Geometry check sheet. Reference: the model listing, model coordinates, mm. Face numbers are marked on the shaded views. A direction names the side the tool comes from. Give positions to 0.01 mm unless a question says otherwise; leave off trailing zeros. Loops run counter-clockwise (first coordinate to the right, second up) from the corner with the lowest first, then second, coordinate; pieces in that order, holes last. Notation, with made-up numbers: (-22, 44.5) -> (37, 44.5) arc R18 ccw to (37, 74.5) -> close; hole circle Ø1 at (54, 16). An arc over 180 degrees is marked (long way). Write item = value, one per line.
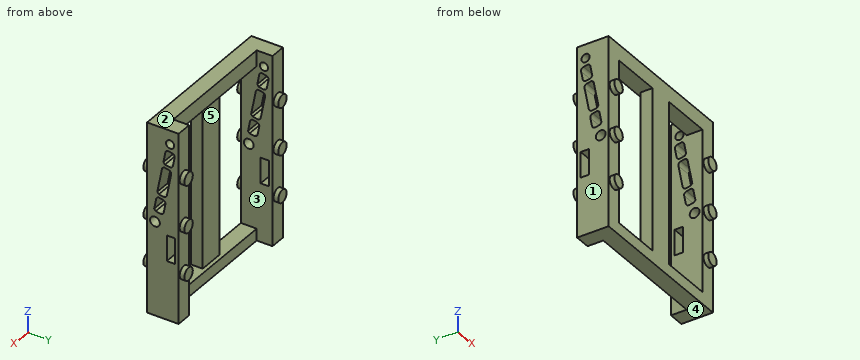
```python
from build123d import *

# Parameters (mm, degrees)
SKETCH1_W               = 100
SKETCH1_H               = 120
SKETCH1_W_2             = 80
SKETCH1_H_2             = 102.5
BOSS_EXTRUDE1_DEPTH     = 20
SKETCH2_R               = 4
BOSS_EXTRUDE2_DEPTH     = 3
MIRROR2_COPY_1_SKETCH_R = 4
MIRROR2_COPY_1_DEPTH    = 3
SKETCH8_W               = 80
SKETCH8_H               = 10
CUT_EXTRUDE5_DEPTH      = 133.018938035
SKETCH12_R              = 3.1
SKETCH12_R_2            = 2.6
CUT_EXTRUDE7_DEPTH      = 14
SKETCH15_W              = 16
SKETCH15_H              = 7.5
BOSS_EXTRUDE4_DEPTH     = 102.5
SKETCH18_W              = 16.2
SKETCH18_H              = 5.2
CUT_EXTRUDE10_DEPTH     = 119.865470175


with BuildPart() as part:
    # Sketch1 → Boss-Extrude1 (new body)
    with BuildSketch(Plane(origin=(0, 0, 0), x_dir=(1, 0, 0), z_dir=(0, 1, 0))):
        Rectangle(SKETCH1_W, SKETCH1_H)
        with Locations((0, 1.25)):
            Rectangle(SKETCH1_W_2, SKETCH1_H_2, mode=Mode.SUBTRACT)
    extrude(amount=BOSS_EXTRUDE1_DEPTH)

    # Sketch2 → Boss-Extrude2 (add)
    with BuildSketch(Plane(origin=(0, 20, 0), x_dir=(1, 0, 0), z_dir=(0, 1, 0))):
        with Locations(Location((-45, 30, 0), (0, 0, 270))):
            Circle(SKETCH2_R)
        with Locations(Location((-45, 0, 0), (0, 0, 270))):
            Circle(SKETCH2_R)
        with Locations(Location((-45, -30, 0), (0, 0, 270))):
            Circle(SKETCH2_R)
    boss_extrude2 = extrude(amount=BOSS_EXTRUDE2_DEPTH)

    # Mirror1: Boss-Extrude2 across plane
    add(boss_extrude2.mirror(Plane(origin=(0, 0, 0), x_dir=(0, 0, 1), z_dir=(1, 0, 0))))

    # Mirror2: Boss-Extrude2 across plane
    add(boss_extrude2.mirror(Plane.ZX.offset(10)))

    # Mirror2 copy 1 sketch → Mirror2 copy 1 (add)
    with BuildSketch(Plane(origin=(0, 0, 0), x_dir=(-1, 0, 0), z_dir=(0, -1, 0))):
        with Locations(Location((-45, 30, 0), (0, 0, 270))):
            Circle(MIRROR2_COPY_1_SKETCH_R)
        with Locations(Location((-45, 0, 0), (0, 0, 270))):
            Circle(MIRROR2_COPY_1_SKETCH_R)
        with Locations(Location((-45, -30, 0), (0, 0, 270))):
            Circle(MIRROR2_COPY_1_SKETCH_R)
    extrude(amount=MIRROR2_COPY_1_DEPTH)

    # Sketch8 → Cut-Extrude5 (cut, through all)
    with BuildSketch(Plane.XY.offset(60)):
        with Locations((0, 15)):
            Rectangle(SKETCH8_W, SKETCH8_H)
    extrude(amount=-CUT_EXTRUDE5_DEPTH, mode=Mode.SUBTRACT)

    # Sketch12 → Cut-Extrude7 (cut)
    with BuildSketch(Plane.ZY.offset(50)):
        with Locations((-0.798318999, 5)):
            Circle(SKETCH12_R)
        with Locations((51.32703264, 14.597276518)):
            Circle(SKETCH12_R_2)
        with BuildLine():
            Line((38.653830619, 10.332015619), (37.447119302, 11.313913997))
            Line((37.447119302, 11.313913997), (36.917785712, 14.071821507))
            ThreePointArc((36.917785712, 14.071821507), (37.226502949, 15.57110114), (38.504949796, 16.412955884))
            Line((38.504949796, 16.412955884), (43.90636018, 17.449665035))
            ThreePointArc((43.90636018, 17.449665035), (45.405639813, 17.140947797), (46.247494557, 15.86250095))
            Line((46.247494557, 15.86250095), (46.812972275, 12.916277104))
            Line((46.812972275, 12.916277104), (45.831073897, 11.709565788))
            Line((45.831073897, 11.709565788), (38.653830619, 10.332015619))
        make_face()
        with BuildLine():
            Line((35.5191142, 10.748612516), (34.953636481, 13.694836362))
            ThreePointArc((34.953636481, 13.694836362), (34.111781738, 14.973283209), (32.612502105, 15.282000446))
            Line((32.612502105, 15.282000446), (18.372420183, 12.548858139))
            ThreePointArc((18.372420183, 12.548858139), (17.093973336, 11.707003396), (16.785256099, 10.207723763))
            Line((16.785256099, 10.207723763), (17.314589689, 7.449816253))
            Line((17.314589689, 7.449816253), (18.521301006, 6.467917875))
            Line((18.521301006, 6.467917875), (34.537215822, 9.5419012))
            Line((34.537215822, 9.5419012), (35.5191142, 10.748612516))
        make_face()
        with BuildLine():
            Line((15.348886072, 7.080929694), (14.783408354, 10.02715354))
            ThreePointArc((14.783408354, 10.02715354), (13.94155361, 11.305600388), (12.442273977, 11.614317625))
            Line((12.442273977, 11.614317625), (7.040863593, 10.577608474))
            ThreePointArc((7.040863593, 10.577608474), (5.762416746, 9.735753731), (5.453699508, 8.236474098))
            Line((5.453699508, 8.236474098), (5.983033099, 5.478566587))
            Line((5.983033099, 5.478566587), (7.189744415, 4.496668209))
            Line((7.189744415, 4.496668209), (14.366987694, 5.874218378))
            Line((14.366987694, 5.874218378), (15.348886072, 7.080929694))
        make_face()
    cut_extrude7 = extrude(amount=-CUT_EXTRUDE7_DEPTH, mode=Mode.SUBTRACT)

    # Mirror5: Cut-Extrude7 across plane
    add(cut_extrude7.mirror(Plane(origin=(0, 0, 0), x_dir=(0, 0, 1), z_dir=(1, 0, 0))), mode=Mode.SUBTRACT)

    # Sketch15 → Boss-Extrude4 (add)
    with BuildSketch(Plane(origin=(0, 0, 50), x_dir=(-1, 0, 0), z_dir=(0, 0, -1))):
        with Locations((0, 3.75)):
            Rectangle(SKETCH15_W, SKETCH15_H)
    extrude(amount=BOSS_EXTRUDE4_DEPTH)

    # Sketch18 → Cut-Extrude10 (cut, through all)
    with BuildSketch(Plane(origin=(50, 0, 0), x_dir=(0, 0, -1), z_dir=(1, 0, 0))):
        with Locations((14.9, 15.1)):
            Rectangle(SKETCH18_W, SKETCH18_H)
    extrude(amount=-CUT_EXTRUDE10_DEPTH, mode=Mode.SUBTRACT)


solid = part.part
```
Item 1: Section check C-C, the plane z = -9.5. Record the cut outline in (x, y).
Answer:
outline = (-50, 0) -> (-40, 0) -> (-40, 12.5) -> (-50, 12.5) -> close; (-50, 17.7) -> (-40, 17.7) -> (-40, 20) -> (-50, 20) -> close; (-8, 0) -> (8, 0) -> (8, 7.5) -> (-8, 7.5) -> close; (40, 0) -> (50, 0) -> (50, 12.5) -> (40, 12.5) -> close; (40, 17.7) -> (50, 17.7) -> (50, 20) -> (40, 20) -> close
Item 2: Gauge pin test, flat ends, axial feed: pin 1 (8 mm diameter, centred on x = 45, z = -16.5, fed in from +Y); pin 2 (11 mm diameter, centred on x = 43, z = -11.5, fed in from -Y); pin 3 (10 mm diameter, centred on y = 7, z = 18, fed in from -X); pin 4 (2 mm diameter, centred on x = -1.5, z = -55, fed in from +Y). Record the tip position at first contact, or that the pin passes through.
Answer:
pin_1 = 20
pin_2 = 0
pin_3 = -50
pin_4 = 10
Item 3: Draft check along X on the marked faces 1, 2 and 3. Enter one of: +X half, -X half, draft (parallel to the pull), parting line (faces both ways), or undercut.
Answer:
face_1 = -X half
face_2 = draft
face_3 = undercut
Item 4: Section check B-B, the plane x = 15.5. Record the cut outline in (y, z).
Answer:
outline = (0, -60) -> (10, -60) -> (10, -52.5) -> (0, -52.5) -> close; (0, 50) -> (10, 50) -> (10, 60) -> (0, 60) -> close
Item 5: Tool access check on the marked faces 4 and 5. Record the directions out of +Z, -Z, +X, -X, +Y, -Y that give a thin tool (end or side, any length) a straight path to the whole face; none if there is none.
Answer:
face_4 = -Z, +X, -X, +Y, -Y
face_5 = +Y
Item 6: Section check A-A, the plane z = -48.5. Record the cut outline in (x, y).
Answer:
outline = (-50, 0) -> (-40, 0) -> (-40, 20) -> (-50, 20) -> close; (-8, 0) -> (8, 0) -> (8, 7.5) -> (-8, 7.5) -> close; (40, 0) -> (50, 0) -> (50, 20) -> (40, 20) -> close
Item 7: Thickness scan on L1, parallel to X at y = 6.75, z = -11.5; L2, parallel to X at y = 19, z = -31; L3, parallel to Z at x = -18, y = 6. Record the ranges inside material, lowest first. Write a range as [from, to].
Answer:
L1 = [-50, -40], [-8, 8], [40, 50]
L2 = [-50, -40], [40, 50]
L3 = [-60, -52.5], [50, 60]
Item 8: Section check D-D, the plane z = -30. Record the cut outline in (x, y), plus the area to 3 significant figures.
Answer:
outline = (-50, 0) -> (-49, 0) -> (-49, -3) -> (-41, -3) -> (-41, 0) -> (-40, 0) -> (-40, 20) -> (-41, 20) -> (-41, 23) -> (-49, 23) -> (-49, 20) -> (-50, 20) -> close; (-8, 0) -> (8, 0) -> (8, 7.5) -> (-8, 7.5) -> close; (40, 0) -> (41, 0) -> (41, -3) -> (49, -3) -> (49, 0) -> (50, 0) -> (50, 20) -> (49, 20) -> (49, 23) -> (41, 23) -> (41, 20) -> (40, 20) -> close
area = 616 mm^2
